from build123d import *

# Parameters (mm, degrees)
F1_R     = 2.578
F1_W     = 72
F1_H     = 143
F2_DEPTH = 3.175
F3_R     = 2
F4_R     = 1


with BuildPart() as f2:
    # F1 (on Front) → F2 (new body)
    with BuildSketch(Plane.XZ):
        Polygon((45.5, 49.5), (45.5, 80.5), (-45.5, 80.5), (-45.5, -80.5), (-5, -80.5), (-5, -77), (5, -77), (5, -80.5), (45.5, -80.5), (45.5, -0.5), (39, -0.5), (39, 49.5), align=None)
        with Locations((-41.444645, -76.658085)):
            Circle(F1_R, mode=Mode.SUBTRACT)
        with Locations((41.444645, -76.658085)):
            Circle(F1_R, mode=Mode.SUBTRACT)
        Rectangle(F1_W, F1_H, mode=Mode.SUBTRACT)
        with Locations((-41.444645, 76.658085)):
            Circle(F1_R, mode=Mode.SUBTRACT)
        with Locations((41.444645, 76.658085)):
            Circle(F1_R, mode=Mode.SUBTRACT)
    extrude(amount=F2_DEPTH)

    # F3
    f3_edges = [f2.edges().sort_by_distance(p)[0] for p in [
        (-36, -1.5875, 71.5),
        (36, -1.5875, 71.5),
        (-45.5, -1.5875, 80.5),
        (45.5, -1.5875, 80.5),
        (45.5, -1.5875, 49.5),
        (39, -1.5875, 49.5),
        (45.5, -1.5875, -0.5),
        (39, -1.5875, -0.5),
        (-36, -1.5875, -71.5),
        (-45.5, -1.5875, -80.5),
        (45.5, -1.5875, -80.5),
        (36, -1.5875, -71.5),
    ]]
    fillet(f3_edges, radius=F3_R)

    # F4
    f4_edges = [f2.edges().sort_by_distance(p)[0] for p in [
        (5, -1.5875, -80.5),
        (5, -1.5875, -77),
        (-5, -1.5875, -77),
        (-5, -1.5875, -80.5),
    ]]
    fillet(f4_edges, radius=F4_R)


solid = f2.part
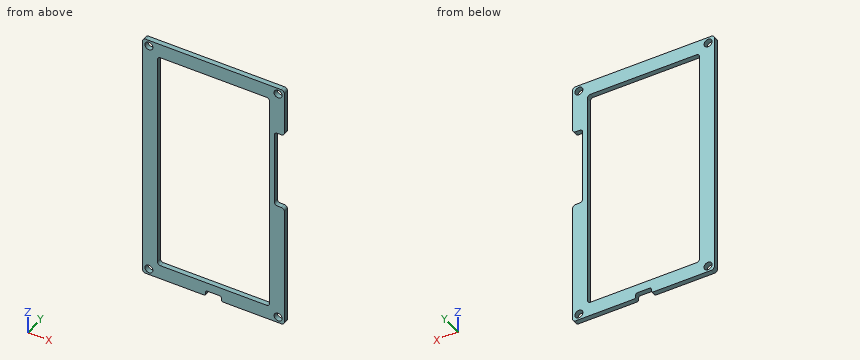
Here's how the part is built. I have some questions about the finished solid (model axes, mm). Round coordinates to 2 decimals unless told otherwise and drop trailing zeros. Order: outer loops, then holes, each group sorted by start corner. A loop starts at its lowest first (then second) coordinate and runs counter-clockwise, first axis right, second up. Notation, with made-up numbers: M 13,72 L 62,72 A18 ccw 62,103 Z; hole C 3.25,26 d10. An arc over 180 degrees is marked long. Return JSON: item names as keys, results as strings. Group by question number.
1. Please list where these lines run through material, in increasing order: probe 1 along Z at (x, y) = (19, -1.55); probe 2 along X at (y, z) = (-2, 23.5); probe 3 along X at (y, z) = (-0.8, 69).
2. If we section it at A-A on x = -28: List the corners of the cut face in (y, z) for me (3 decimals), then the cut area to 4 significant figures.
3. If we section it at B-B on z = -65: List the corners of the cut face in (x, y) for me (3 decimals), then the cut area to 3 significant figures.
4. If we section it at C-C on y = -2.65: State how many separate pieces and enclosed holes the cut face has, then the cut area to 3 significant figures.
5. I'm going to push flat-ended pins straight in: pin 1 Ø6.5 at (x, z) = (-41.44, 76.66) entering from +Y; pin 2 Ø0.8 at (y, z) = (-2, -79) entering from +X; pin 3 Ø0.8 at (y, z) = (-2, -79) entering from -X. Where does each tip first touch, or does it pass through?
Reply:
{
 "1": {"probe 1": "-80.5 to -71.5, 71.5 to 80.5", "probe 2": "-45.5 to -36, 36 to 39", "probe 3": "-45.5 to -36, 36 to 45.5"},
 "2": {"outline": "M -3.175,-80.5 L 0,-80.5 L 0,-71.5 L -3.175,-71.5 Z; M -3.175,71.5 L 0,71.5 L 0,80.5 L -3.175,80.5 Z", "area": "57.15 mm^2"},
 "3": {"outline": "M -45.5,-3.175 L -36,-3.175 L -36,0 L -45.5,0 Z; M 36,-3.175 L 45.5,-3.175 L 45.5,0 L 36,0 Z", "area": "60.3 mm^2"},
 "4": {"separate pieces": "1", "enclosed holes": "5", "area": "3,910 mm^2"},
 "5": {"pin 1": "y = 0", "pin 2": "x = 45.5", "pin 3": "x = -45.5"}
}
